Input: part model. Units: mm. Frame: model coordinates. Face numbers are marked on the shaded views. A direction names the side the tool comes from. Coordinates: 2 decimals unless noted, no trailing zeros. Loops run counter-clockwise (first coordinate to the right, second up) from the corner with the lowest first, then second, coordinate; pieces in that order, holes last.
(1) Mould query, pull axis X, two halves, no side actions, for the marked faces 3, 4, 5 and 6. Classes: released by +X, released by -X, zero draft, split by the parting line, or undercut.
(2) Set-up query: the marked faces 1 and 2. Return all of +Z, -Z, +X, -X, +Y, -Y with unobstructed straight access to the full face (end or side cutting, diameter ignored); none if empty.
(3) Section A-A, the plane y = 0. Return loops of the section in (x, z) (3 decimals), then the cut area to 3 significant figures.
(4) Section D-D, the plane x = -9.25. Return loops of the section in (y, z), then the cut area to 3 significant figures.
(5) Section B-B, the plane x = 0. Return loops of the section in (y, z) (1 decimal).
(6) Line query: L1, parallel to X at y = -5.25, z = 3.25; L2, parallel to Y at x = 0, z = 1.35 (1 decimal); L3, parallel to X at y = -3.75, z = 0.5. Output: solid intervals per line, ascending.
(7) Contact query for flat-ended pins moving along their axis: P1, Ø3, axis at y = 9.5, z = 5, coming from the +X side; P2, Ø4, axis at x = -3.5, z = 4.5, coming from the +Y side; P3, Ø2, axis at x = -8, z = 4, coming from the -Y side. Output: stop coordinate, or through.
(8) Section C-C, the plane z = 1.5. Give the number of separate pieces and of enclosed holes in the cut face, then the cut area to 3 significant figures.
```python
from build123d import *

# Parameters (mm, degrees)
SKETCH1_R           = 12.7
SKETCH1_R_2         = 1.5875
BOSS_EXTRUDE1_DEPTH = 5.08
SKETCH2_R           = 5.969
BOSS_EXTRUDE2_DEPTH = 4.191
SKETCH3_R           = 3.175
CUT_EXTRUDE1_DEPTH  = 9.271


with BuildPart() as part:
    # Sketch1 → Boss-Extrude1 (new body)
    with BuildSketch(Plane.XY):
        Circle(SKETCH1_R)
        with Locations((0, 9.525)):
            Circle(SKETCH1_R_2, mode=Mode.SUBTRACT)
        with Locations((8.248891971, 4.7625)):
            Circle(SKETCH1_R_2, mode=Mode.SUBTRACT)
        with Locations((8.248891971, -4.7625)):
            Circle(SKETCH1_R_2, mode=Mode.SUBTRACT)
        with Locations((0, -9.525)):
            Circle(SKETCH1_R_2, mode=Mode.SUBTRACT)
        with Locations((-8.248891971, -4.7625)):
            Circle(SKETCH1_R_2, mode=Mode.SUBTRACT)
        with Locations((-8.248891971, 4.7625)):
            Circle(SKETCH1_R_2, mode=Mode.SUBTRACT)
    extrude(amount=BOSS_EXTRUDE1_DEPTH)

    # Sketch2 → Boss-Extrude2 (add)
    with BuildSketch(Plane.XY.offset(5.08)):
        Circle(SKETCH2_R)
    extrude(amount=BOSS_EXTRUDE2_DEPTH)

    # Sketch3 → Cut-Extrude1 (cut)
    with BuildSketch(Plane.XY.offset(9.271)):
        Circle(SKETCH3_R)
    extrude(amount=-CUT_EXTRUDE1_DEPTH, mode=Mode.SUBTRACT)


solid = part.part
```
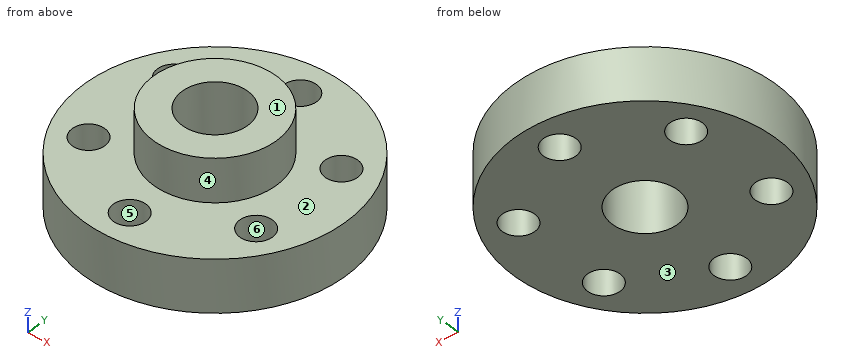
Report:
1. face 3: zero draft
1. face 4: split by the parting line
1. face 5: undercut
1. face 6: undercut
2. face 1: +Z, +X, -X, +Y, -Y
2. face 2: +Z
3. outline: (-12.7, 0) - (-3.175, 0) - (-3.175, 9.271) - (-5.969, 9.271) - (-5.969, 5.08) - (-12.7, 5.08) - close; (3.175, 0) - (12.7, 0) - (12.7, 5.08) - (5.969, 5.08) - (5.969, 9.271) - (3.175, 9.271) - close
3. area: 120 mm2
4. outline: (-8.7, 0) - (-5.99, 0) - (-5.99, 5.08) - (-8.7, 5.08) - close; (-3.53, 0) - (3.53, 0) - (3.53, 5.08) - (-3.53, 5.08) - close; (5.99, 0) - (8.7, 0) - (8.7, 5.08) - (5.99, 5.08) - close
4. area: 63.4 mm2
5. outline: (-12.7, 0) - (-11.1, 0) - (-11.1, 5.1) - (-12.7, 5.1) - close; (-7.9, 0) - (-3.2, 0) - (-3.2, 9.3) - (-6, 9.3) - (-6, 5.1) - (-7.9, 5.1) - close; (3.2, 0) - (7.9, 0) - (7.9, 5.1) - (6, 5.1) - (6, 9.3) - (3.2, 9.3) - close; (11.1, 0) - (12.7, 0) - (12.7, 5.1) - (11.1, 5.1) - close
6. L1: x = -11.56 to -9.76, -6.74 to 6.74, 9.76 to 11.56
6. L2: y = -12.7 to -11.1, -7.9 to -3.2, 3.2 to 7.9, 11.1 to 12.7
6. L3: x = -12.13 to -9.47, -7.03 to 7.03, 9.47 to 12.13
7. P1: stops at x = 9.86
7. P2: stops at y = 12.61
7. P3: stops at y = -10.6
8. separate pieces: 1
8. enclosed holes: 7
8. area: 428 mm2
